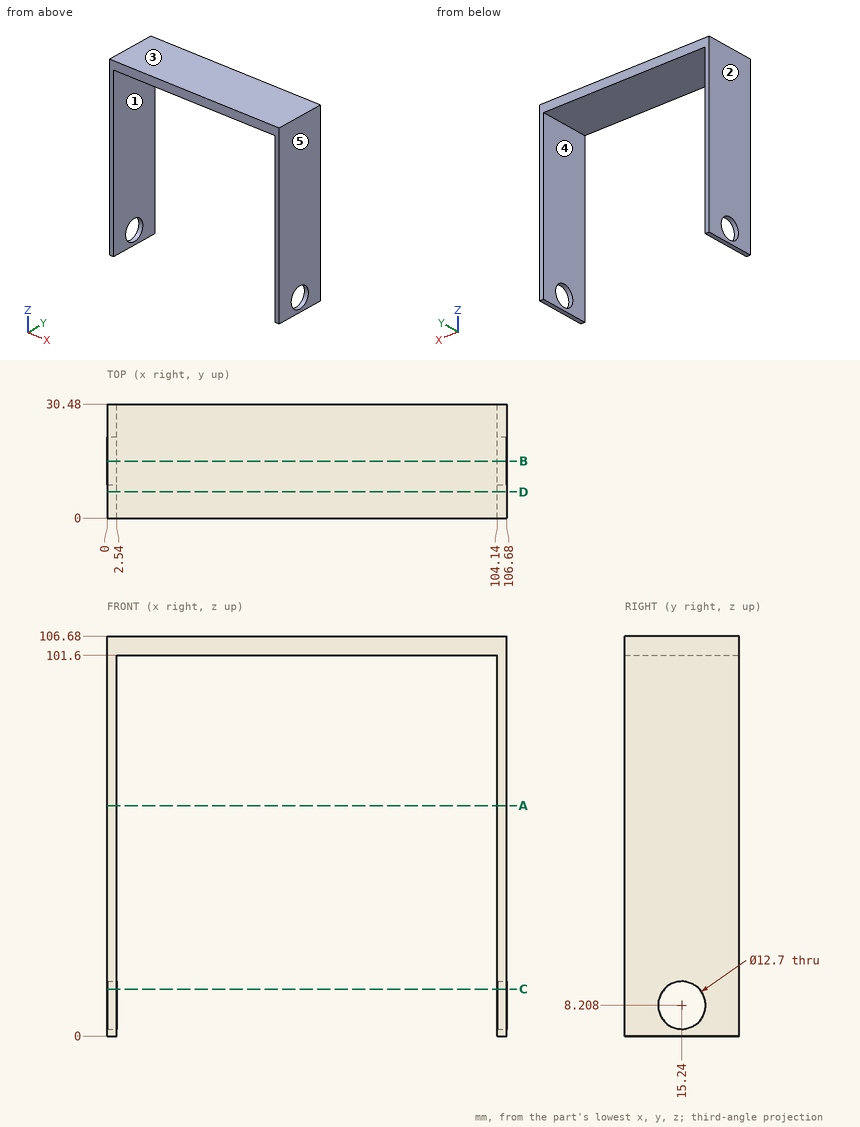
Here's the drawing with two shaded views (mm, measured from the low corner). I have some questions. A direction names the side the tool comes from. Coordinates: 2 decimals unless noted, no trailing zeros. Write each loop counter-clockwise with the first axis right and the second up, starting at its lowest first coordinate (ties: lowest second). Pieces come first, ordered by that corner, then holes. Notation, with made-up numbers: (17.5, -19.75) -> (61.5, -19.75) arc R18 ccw to (61.5, 12.25) -> close; hole circle Ø5 at (86, 88). An arc over 180 degrees is marked (long way). Answer as CSV lines item,"result".
1) Will these pins go through, and if not, where does the flat tip stop? P1, Ø1, axis at x = 71.5, y = 23, coming from the -Z side; P2, Ø7.5, axis at y = 15.24, z = 8.21, coming from the -X side.
Check result:
P1,"z = 101.6"
P2,"through"
2) If we section it at A-A on z = 61.5: Please give me the cut outline in (x, y), then the cut area to 3 significant figures.
Check result:
outline,"(0, 0) -> (2.54, 0) -> (2.54, 30.48) -> (0, 30.48) -> close; (104.14, 0) -> (106.68, 0) -> (106.68, 30.48) -> (104.14, 30.48) -> close"
area,"155 mm²"
3) On a 3-axis mill with a long thin cutter (end or side, diameter ignored), from which of +Z, -Z, +X, -X, +Y, -Y can I reach the whole of each face in a straight line? I mean the marked faces 1 and 2. Say none if no direction works.
Check result:
face 1,"-Z, +Y, -Y"
face 2,"+Z, -Z, -X, +Y, -Y"
4) If we section it at B-B on y = 15.24: Please give me the cut outline in (x, z).
Check result:
outline,"(0, 0) -> (2.54, 0) -> (2.54, 1.86) -> (0, 1.86) -> close; (0, 14.56) -> (2.54, 14.56) -> (2.54, 101.6) -> (104.14, 101.6) -> (104.14, 14.56) -> (106.68, 14.56) -> (106.68, 106.68) -> (0, 106.68) -> close; (104.14, 0) -> (106.68, 0) -> (106.68, 1.86) -> (104.14, 1.86) -> close"
5) If we section it at C-C on z = 12.5: Please give me the cut outline in (x, y), then the cut area to 3 significant figures.
Check result:
outline,"(0, 0) -> (2.54, 0) -> (2.54, 10.56) -> (0, 10.56) -> close; (0, 19.92) -> (2.54, 19.92) -> (2.54, 30.48) -> (0, 30.48) -> close; (104.14, 0) -> (106.68, 0) -> (106.68, 10.56) -> (104.14, 10.56) -> close; (104.14, 19.92) -> (106.68, 19.92) -> (106.68, 30.48) -> (104.14, 30.48) -> close"
area,"107 mm²"
6) If we mould it in two halves opening along X, with no side actions, what happens to the marked faces 3, 4 and 5? For each: +X half, -X half, draft (parallel to the pull), parting line (faces both ways), or undercut.
Check result:
face 3,"draft"
face 4,"undercut"
face 5,"+X half"
7) If we section it at D-D on y = 7: Please give me the cut outline in (x, z).
Check result:
outline,"(0, 0) -> (2.54, 0) -> (2.54, 101.6) -> (104.14, 101.6) -> (104.14, 0) -> (106.68, 0) -> (106.68, 106.68) -> (0, 106.68) -> close"
8) If I drill on line 1 (X direction, y = 27, z = 101); line 2 (Z direction, x = 105.05, y = 15.24); line 3 (Z direction, x = 94, y = 9.5), over which ranges is the centre line in solid material (lowest first)? Write a range as from..to.
Check result:
line 1,"0..2.54, 104.14..106.68"
line 2,"0..1.86, 14.56..106.68"
line 3,"101.6..106.68"
